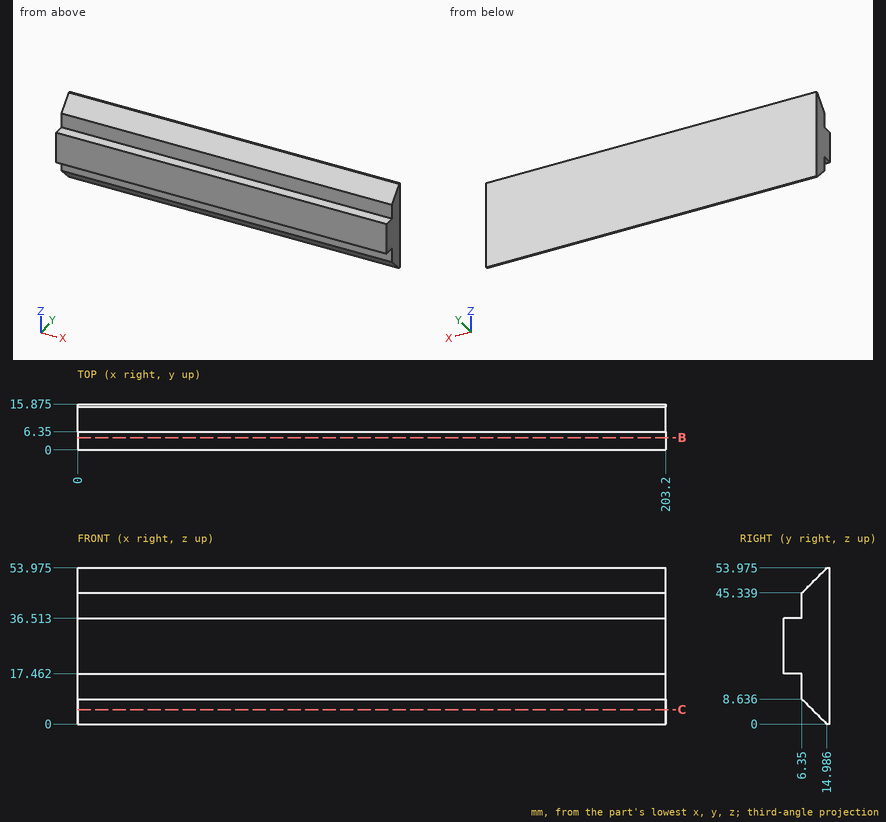
Source: three-view drawing plus pictorial views. Frame: mm from the lowest corner of the part. Give positions to 0.01 mm unless a question says otherwise; leave off trailing zeros. Loops run counter-clockwise (first coordinate to the right, second up) from the corner with the lowest first, then second, coordinate; pieces in that order, holes last.
1) Contact query for flat-ended pins moving along their axis: pin 1 (5 mm diameter, centred on x = 23.5, z = 33.5, fed in from -Y); pin 2 (3 mm diameter, centred on x = 162, y = 5.5, fed in from +Z); pin 3 (3 mm diameter, centred on x = 162.5, y = 6, fed in from -Z) (1 decimal); pin 4 (6 mm diameter, centred on x = 137, y = 7.5, fed in from +Z). Output: stop coordinate, or through.
A:
pin 1: stops at y = 0
pin 2: stops at z = 45.99
pin 3: stops at z = 7.5
pin 4: stops at z = 49.49
2) Section query C-C on z = 5. Return the cut outline in (x, y) (1 decimal), and give its area (3 significant figures).
A:
outline: (0, 10) - (203.2, 10) - (203.2, 15.9) - (0, 15.9) - close
area: 1,200 mm2
3) Section query B-B on y = 4.25. Return the cut outline in (x, z).
A:
outline: (0, 17.46) - (203.2, 17.46) - (203.2, 36.51) - (0, 36.51) - close
4) Line query: L1, parallel to Z at x = 138, y = 5; L2, parallel to Y at x = 94, z = 3.5 (1 decimal); L3, parallel to Y at x = 181, z = 5.5 (1 decimal). Output: solid intervals per line, ascending.
A:
L1: z = 17.46 to 36.51
L2: y = 11.5 to 15.9
L3: y = 9.5 to 15.9
